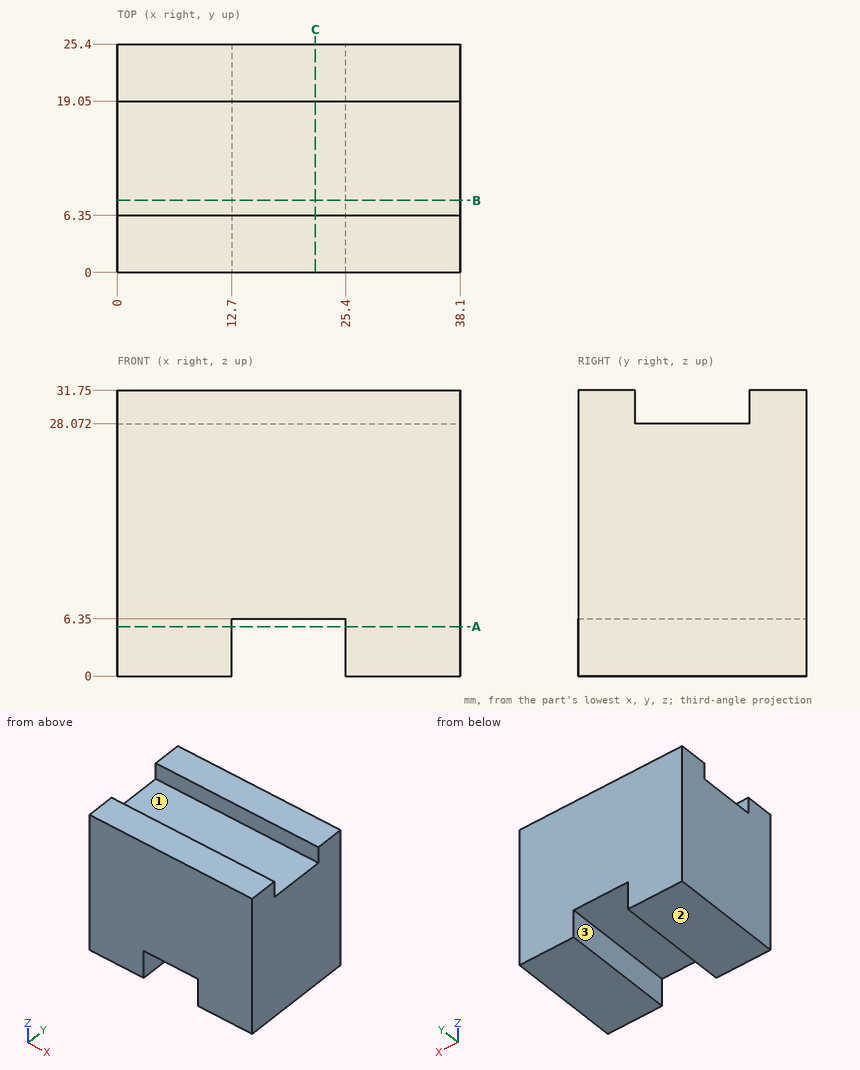
Geometry check sheet. Reference: drawing and pictorial views, mm from the part's lowest x, y, z. A direction names the side the tool comes from. Round coordinates to 2 decimals unless told otherwise and drop trailing zeros. Loops run counter-clockwise (first coordinate to the right, second up) from the corner with the lowest first, then second, coordinate; pieces in that order, holes last. Notation, with made-up numbers: (86.5, 2.5) - (123.5, 2.5) arc R27 ccw to (123.5, 26.5) - close; hole circle Ø4 at (72, 50.25). An arc over 180 degrees is marked (long way). Answer as CSV lines item,"result".
(1) Material ranges on line 1 along Z through (x, y) = (12.5, 9.75); line 2 along Z through (x, y) = (14, 6.25), recorded low to high.
Output values:
line 1,"z = 0 to 28.07"
line 2,"z = 6.35 to 31.75"
(2) Cross-section at C-C, the plane x = 22. Enter the section's corners in (y, z).
Output values:
outline,"(0, 6.35) - (25.4, 6.35) - (25.4, 31.75) - (19.05, 31.75) - (19.05, 28.07) - (6.35, 28.07) - (6.35, 31.75) - (0, 31.75) - close"
(3) Set-up check for the marked faces 1, 2 and 3: record each of +Z, -Z, +X, -X, +Y, -Y from which the full face is reachable in a straight line by a thin tool's end or side.
Output values:
face 1,"+Z, +X, -X"
face 2,"-Z, +X, -X, +Y, -Y"
face 3,"-Z, +Y, -Y"
(4) Cross-section at A-A, the plane z = 5.5. Enter the section's corners in (x, y).
Output values:
outline,"(0, 0) - (12.7, 0) - (12.7, 25.4) - (0, 25.4) - close; (25.4, 0) - (38.1, 0) - (38.1, 25.4) - (25.4, 25.4) - close"
(5) Cross-section at B-B, the plane y = 8. Enter the section's corners in (x, z), and give its area (3 significant figures).
Output values:
outline,"(0, 0) - (12.7, 0) - (12.7, 6.35) - (25.4, 6.35) - (25.4, 0) - (38.1, 0) - (38.1, 28.07) - (0, 28.07) - close"
area,"989 mm²"
